Part model, mm, in its own coordinate system. Face numbers are marked on the shaded views. A direction names the side the tool comes from. Round coordinates to 2 decimals unless told otherwise and drop trailing zeros. Write each loop counter-clockwise with the first axis right and the second up, starting at its lowest first coordinate (ties: lowest second). Pieces come first, ordered by that corner, then holes.
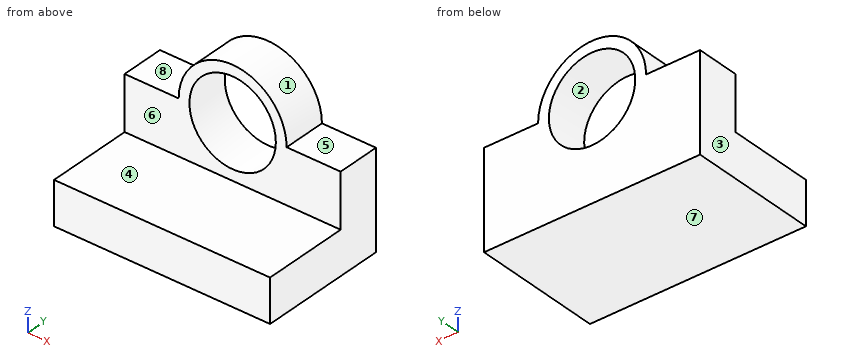
Autodesk Fusion 360 part; units mm, degrees
sketch "Sketch1" plane through (0, 0, 0) normal (0, 1, 0) x (1, 0, 0)
  line L0 (-50, -10) -> (50, -10)
  line L1 (50, -10) -> (50, -55)
  line L2 (50, -55) -> (-50, -55)
  line L3 (-50, -55) -> (-50, -10)
  circle A0 centre (0, -55) radius 20
  circle A1 centre (0, -55) radius 25
  dimension "d1" = 100
  dimension "d2" = 45
  dimension "d4" = 50
extrude "Extrude1" add sketch "Sketch1" along normal blind 20 contours L0 L1 L2 L3 A1 | L2 A0 A1 | L2 A0 A1
sketch "Sketch2" plane through (0, 0, 10) normal (0, 0, -1) x (1, 0, 0)
  line L0 (50, 0) -> (-50, 0)
  line L1 (-50, 0) -> (-50, -20)
  line L2 (-50, -20) -> (50, -20)
  line L3 (50, -20) -> (50, 0)
  line L4 (-50, 0) -> (-50, 40)
  line L5 (-50, 40) -> (50, 40)
  line L6 (50, 40) -> (50, 0)
  dimension "d7" = 40
extrude "Extrude2" add sketch "Sketch2" against normal blind 20 contours L0 L4 L5 L6
Q1. Wall check: line 1 (Z direction, x = 0, y = 8); line 2 (Y direction, x = 23, z = 63); line 3 (Z direction, x = 16, y = -1.5). Give the ranges that are in metal, low to high.
Q2. Two-plate mould, pull along X, no slides. Class the marked faces 1, 2, 3 and 4: released by +X, released by -X, zero draft, split by the parting line, or undercut.
Q3. Saw through at A-A, the plane z = 57. Write the cut outline in (x, y).
Q4. Tool access for the marked faces 5, 6, 7 and 8: list every direction of +Z, -Z, +X, -X, +Y, -Y with a clear straight run to the whole face (end or side of a thin tool).
Q5. Saw through at C-C, the plane x = 43.5. Write the cut outline in (y, z), and give its area (3 significant figures).
Q6. Saw through at B-B, the plane x = 0. Write the cut outline in (y, z), and give its area (3 significant figures).
Q7. Drop flat-ended pins along their axis: P1, Ø10, axis at x = 15.5, y = -3.5, coming from the +Z side; P2, Ø20, axis at x = -8, y = -19.5, coming from the +Z side; P3, Ø15, axis at x = -19.5, z = 56, coming from the -Y side. Give the stop position or say it passes through.
Q8. Saw through at D-D, the plane z = 44. Write the cut outline in (x, y), and give its area (3 significant figures).
Computed:
1. line 1: z = 10 to 35, 75 to 80
1. line 2: y = 0 to 20
1. line 3: z = 10 to 30
2. face 1: split by the parting line
2. face 2: undercut
2. face 3: released by -X
2. face 4: zero draft
3. outline: (-24.92, 0) - (-19.9, 0) - (-19.9, 20) - (-24.92, 20) - close; (19.9, 0) - (24.92, 0) - (24.92, 20) - (19.9, 20) - close
4. face 5: +Z, +X, +Y, -Y
4. face 6: +Z, +X, -X, -Y
4. face 7: -Z, +X, -X, +Y, -Y
4. face 8: +Z, -X, +Y, -Y
5. outline: (-40, 10) - (20, 10) - (20, 55) - (0, 55) - (0, 30) - (-40, 30) - close
5. area: 1,700 mm2
6. outline: (-40, 10) - (20, 10) - (20, 35) - (0, 35) - (0, 30) - (-40, 30) - close; (0, 75) - (20, 75) - (20, 80) - (0, 80) - close
6. area: 1,400 mm2
7. P1: stops at z = 76.97
7. P2: stops at z = 30
7. P3: stops at y = 0
8. outline: (-50, 0) - (-16.7, 0) - (-16.7, 20) - (-50, 20) - close; (16.7, 0) - (50, 0) - (50, 20) - (16.7, 20) - close
8. area: 1,330 mm2
